Work out the finished part from the listing and answer in its coordinate system (mm). A direction names the side the tool comes from. Round coordinates to 2 decimals unless told otherwise and drop trailing zeros. Order: outer loops, then holes, each group sorted by start corner. A loop starts at its lowest first (then second) coordinate and runs counter-clockwise, first axis right, second up. Notation, with made-up numbers: (19, -39.5) - (32, -39.5) arc R21 ccw to (32, -31.5) - close; hole circle Ø5 at (72, 89.25). An arc over 180 degrees is marked (long way). Put each result on its own line as item: value.
```python
from build123d import *

# Parameters (mm, degrees)
F1_DEPTH  = 40
F2_R      = 15
F3_DEPTH  = 90
F4_R      = 30
F5_DEPTH  = 25
F6_R      = 8
F7_DEPTH  = 6
F10_DEPTH = 10
F11_R     = 6
F12_DEPTH = 10
F13_R     = 15
F14_DEPTH = 85.001
F15_R     = 6
F16_DEPTH = 8
F17_R     = 7.5
F18_DEPTH = 110


# Not quite as in the source:
# - a pattern or mirror of a feature is missing from the dataset's text; its kind, count and spacing are read off the source's solid


with BuildPart() as f1:
    # F0 (on Front) → F1 (new body)
    with BuildSketch(Plane.XZ):
        Polygon((15, 20), (-15, 20), (-20, -20), (20, -20), align=None)
    extrude(amount=-F1_DEPTH)

    # F2 (on face) → F3 (join)
    with BuildSketch(Plane(origin=(0, 40, 0), x_dir=(-1, 0, 0), z_dir=(0, 1, 0))):
        Circle(F2_R)
    extrude(amount=F3_DEPTH)

    # F4 (on Top) → F5 (join, symmetric)
    with BuildSketch(Plane.XY):
        with Locations((0, 130)):
            Circle(F4_R)
    extrude(amount=F5_DEPTH, both=True)

    # F6 (on Right) → F7 (join, symmetric)
    with BuildSketch(Plane.YZ):
        with BuildLine():
            Line((40, 44), (40, 10.4397451505))
            Line((40, 10.4397451505), (40, 6.8427645601))
            Line((40, 6.8427645601), (80, 6.8427645601))
            Line((80, 6.8427645601), (80, 44))
            ThreePointArc((80, 44), (60, 64), (40, 44))
        make_face()
        with Locations((60, 44)):
            Circle(F6_R, mode=Mode.SUBTRACT)
    extrude(amount=F7_DEPTH, both=True)

    # F9 (on offset) → F10 (join)
    with BuildSketch(Plane.YZ.offset(15)):
        with BuildLine():
            Line((0, -20), (5.2618519826, -47.7905184139))
            ThreePointArc((5.2618519826, -47.7905184139), (20, -60), (34.7381480174, -47.7905184139))
            Line((34.7381480174, -47.7905184139), (40, -20))
            Line((40, -20), (0, -20))
        make_face()
    f10 = extrude(amount=-F10_DEPTH)

    # F10_copies: F10 across plane
    add(f10.mirror(Plane(origin=(0, 0, 0), x_dir=(0, 0, -1), z_dir=(-1, 0, 0))))

    # F11 (on face) → F12 (cut, through all)
    with BuildSketch(Plane.YZ.offset(15)):
        with Locations((20, -45)):
            Circle(F11_R)
    f12 = extrude(amount=-F12_DEPTH, mode=Mode.SUBTRACT)

    # F12_copies: F12 across plane
    add(f12.mirror(Plane(origin=(0, 0, 0), x_dir=(0, 0, -1), z_dir=(-1, 0, 0))), mode=Mode.SUBTRACT)

    # F13 (on face) → F14 (cut, through all)
    with BuildSketch(Plane.XY.offset(25)):
        with Locations((0, 130)):
            Circle(F13_R)
    extrude(amount=-F14_DEPTH, mode=Mode.SUBTRACT)

    # F15 (on face) → F16 (cut)
    with BuildSketch(Plane.XY.offset(20)):
        with Locations((0, 20)):
            Circle(F15_R)
    extrude(amount=-F16_DEPTH, mode=Mode.SUBTRACT)

    # F17 (on face) → F18 (cut)
    with BuildSketch(Plane.XZ):
        Circle(F17_R)
    extrude(amount=-F18_DEPTH, mode=Mode.SUBTRACT)


solid = f1.part
```
1) A cutting plane is placed at D-D on y = 60. Write down the section's boundary in (x, z).
Findings below:
outline: (-6, 13.75) arc R15 ccw (long way) to (6, 13.75) - (6, 36) - (-6, 36) - close; (-6, 52) - (6, 52) - (6, 64) - (-6, 64) - close; hole circle Ø15 at (0, 0)
2) Straight lines are drawn through the part: L1, parallel to Y at x = 0.5, z = 13; L2, parallel to Y at x = 0, z = 7; L3, parallel to Y at x = 0, z = 9. For each, find the intervals that lie inside material, in ascending order. Write a range as from..to.
Findings below:
L1: y = 0..14.02, 25.98..115.01, 144.99..160
L2: y = 110..115, 145..160
L3: y = 0..115, 145..160
3) For faces 1 (the flat face through (-6, 60, 34)), 2 (the flat face through (15, 20, -35)), 3 (the flat face through (-15, 20, -35)), 4 (the flat face through (17.535, 19.72, -0.28)), determine the directions among +Z, -Z, +X, -X, +Y, -Y from which every point of the face is accessible in a straight line to the end or side of a thin tool.
Findings below:
face 1: +Z, -X
face 2: -Z, +X, -Y
face 3: -Z, -X, -Y
face 4: +Z, +X, -Y
4) A cutting plane is placed at C-C on y = 130. Write down the section's boundary in (x, z), then the cut area to 3 significant figures.
Findings below:
outline: (-30, -25) - (-15, -25) - (-15, 25) - (-30, 25) - close; (15, -25) - (30, -25) - (30, 25) - (15, 25) - close
area: 1,500 mm2
5) Given pin 1 Ø4 at (x, y) = (13.5, 106) entering from -Z; pin 2 Ø5 at (x, y) = (0, 15) entering from -Z; pin 3 Ø12 at (x, z) = (-11.5, 27) entering from +Y; pin 4 Ø17 at (x, z) = (0, 0) entering from -Y, each flat-ended and moving along its own axis, determine where each tip first touches the part or whether it passes through.
Findings below:
pin 1: stops at z = -25
pin 2: stops at z = -20
pin 3: stops at y = 159.43
pin 4: stops at y = 0
6) A cutting plane is placed at A-A on x = 0. Write down the section's boundary in (y, z), then the cut area to 3 significant figures.
Findings below:
outline: (0, -20) - (40, -20) - (40, -15) - (100, -15) - (100, -25) - (115, -25) - (115, 25) - (100, 25) - (100, 15) - (80, 15) - (80, 44) arc R20 ccw to (40, 44) - (40, 20) - (26, 20) - (26, 12) - (14, 12) - (14, 20) - (0, 20) - (0, 7.5) - (110, 7.5) - (110, -7.5) - (0, -7.5) - close; (145, -25) - (160, -25) - (160, 25) - (145, 25) - close; hole circle Ø16 at (60, 44)
area: 4,740 mm2
7) For a pull along Z with two mould halves and no side action, classify faces 5 (the flat face through (10.07, 2.594, -33.701)), 6 (the flat face through (6, 60, 34)), 7 (the cylindrical face through (-7.493, 54.23, 0.33)), 8 (the flat face through (-17.465, 19.72, 0.28)) as pulls with the +Z half, pulls with the -Z half, needs draft (parallel to the pull), parting line crosses it, or undercut.
Findings below:
face 5: pulls with the -Z half
face 6: needs draft
face 7: undercut
face 8: pulls with the +Z half
8) A cutting plane is placed at B-B on y = 20. Write down the section's boundary in (x, z).
Findings below:
outline: (-20, -20) - (-15, -20) - (-15, -39) - (-5, -39) - (-5, -20) - (5, -20) - (5, -39) - (15, -39) - (15, -20) - (20, -20) - (15, 20) - (6, 20) - (6, 12) - (-6, 12) - (-6, 20) - (-15, 20) - close; (-15, -60) - (-5, -60) - (-5, -51) - (-15, -51) - close; (5, -60) - (15, -60) - (15, -51) - (5, -51) - close; hole circle Ø15 at (0, 0)
